The model under review builds one solid part; all positions refer to its coordinate system, in mm. A direction names the side the tool comes from. Round coordinates to 2 decimals unless told otherwise and drop trailing zeros. Order: outer loops, then holes, each group sorted by start corner. A loop starts at its lowest first (then second) coordinate and runs counter-clockwise, first axis right, second up. Notation, with made-up numbers: M 12.5,52 L 30.5,52 A22 cw 30.5,79 Z; hole C -30.75,68.5 d10. An arc over 180 degrees is marked long. Answer as a JSON object with one key per item and string values. Group by question number.
1) To check wall thickness, follow line 1 (Y direction, x = -23.25, z = 0); line 2 (X direction, y = -72, z = -17); line 3 (Z direction, x = -4.5, y = 14.5). State the ranges of each line that lie inside material, in increasing order.
2) Consider section C-C, the plane y = 69.85. Write out the cut boundary in (x, z).
3) Consider section B-B, the plane y = -11.5. Write out the cut boundary in (x, z).
4) Consider section A-A, the plane z = 0. Write out the cut boundary in (x, y).
5) Consider section D-D, the plane x = 10.5. Write out the cut boundary in (y, z), then the cut area to 3 significant figures.
6) For faces 5 (the flat face through (0, 1, -19.05)), 6 (the cylindrical face through (-23.49, 1.42, 23.59)), list the 3-axis set-ups (+Z, -Z, +X, -X, +Y, -Y) from which the entire face can be reached by the end or side of a thin tool; tool diameter is ignored.
7) The part is to be moulded in two halves that separate along Y. For faces 1 (the flat face through (0, -101.6, 22)), 2 (the cylindrical face through (22.27, 54.23, 3.47)), 3 (the cylindrical face through (-22.18, 54.23, 3.47)), 4 (the flat face through (-25.4, 1, 0)), say which applies: +Y half, -Y half, draft (parallel to the pull), parting line (faces both ways), or undercut.
```python
from build123d import *

# Parameters (mm, degrees)
BOSS_EXTRUDE1_DEPTH = 101.6
SKETCH2_R           = 16.002
CUT_EXTRUDE1_DEPTH  = 51.8


with BuildPart() as part:
    # Sketch1 → Boss-Extrude1 (new body, symmetric)
    with BuildSketch(Plane(origin=(0, 0, 0), x_dir=(0, 0, -1), z_dir=(0, 1, 0))):
        with BuildLine():
            Line((-19.05, 25.4), (19.05, 25.4))
            ThreePointArc((19.05, 25.4), (23.540128061, 23.540128061), (25.4, 19.05))
            Line((25.4, 19.05), (25.4, -19.05))
            ThreePointArc((25.4, -19.05), (23.540128061, -23.540128061), (19.05, -25.4))
            Line((19.05, -25.4), (-19.05, -25.4))
            ThreePointArc((-19.05, -25.4), (-23.540128061, -23.540128061), (-25.4, -19.05))
            Line((-25.4, -19.05), (-25.4, 19.05))
            ThreePointArc((-25.4, 19.05), (-23.540128061, 23.540128061), (-19.05, 25.4))
        make_face()
        with BuildLine():
            Line((-16.66875, 19.05), (16.66875, 19.05))
            ThreePointArc((16.66875, 19.05), (18.352548023, 18.352548023), (19.05, 16.66875))
            Line((19.05, 16.66875), (19.05, -16.66875))
            ThreePointArc((19.05, -16.66875), (18.352548023, -18.352548023), (16.66875, -19.05))
            Line((16.66875, -19.05), (-16.66875, -19.05))
            ThreePointArc((-16.66875, -19.05), (-18.352548023, -18.352548023), (-19.05, -16.66875))
            Line((-19.05, -16.66875), (-19.05, 16.66875))
            ThreePointArc((-19.05, 16.66875), (-18.352548023, 18.352548023), (-16.66875, 19.05))
        make_face(mode=Mode.SUBTRACT)
    extrude(amount=BOSS_EXTRUDE1_DEPTH, both=True)

    # Sketch2 → Cut-Extrude1 (cut, through all)
    with BuildSketch(Plane(origin=(25.4, 0, 0), x_dir=(0, 0, -1), z_dir=(1, 0, 0))):
        with Locations((0, 69.85)):
            Circle(SKETCH2_R)
    extrude(amount=-CUT_EXTRUDE1_DEPTH, mode=Mode.SUBTRACT)


solid = part.part
```
Results list:
{
 "1": {"line 1": "-101.6 to 53.85, 85.85 to 101.6", "line 2": "-25.4 to -19.03, 19.03 to 25.4", "line 3": "-25.4 to -19.05, 19.05 to 25.4"},
 "2": {"outline": "M -25.4,-19.05 A6.35 ccw -19.05,-25.4 L 19.05,-25.4 A6.35 ccw 25.4,-19.05 L 25.4,-16 L 19.05,-16 L 19.05,-16.67 A2.38 cw 16.67,-19.05 L -16.67,-19.05 A2.38 cw -19.05,-16.67 L -19.05,-16 L -25.4,-16 Z; M -25.4,16 L -19.05,16 L -19.05,16.67 A2.38 cw -16.67,19.05 L 16.67,19.05 A2.38 cw 19.05,16.67 L 19.05,16 L 25.4,16 L 25.4,19.05 A6.35 ccw 19.05,25.4 L -19.05,25.4 A6.35 ccw -25.4,19.05 Z"},
 "3": {"outline": "M -25.4,-19.05 A6.35 ccw -19.05,-25.4 L 19.05,-25.4 A6.35 ccw 25.4,-19.05 L 25.4,19.05 A6.35 ccw 19.05,25.4 L -19.05,25.4 A6.35 ccw -25.4,19.05 Z; hole M -19.05,-16.67 A2.38 ccw -16.67,-19.05 L 16.67,-19.05 A2.38 ccw 19.05,-16.67 L 19.05,16.67 A2.38 ccw 16.67,19.05 L -16.67,19.05 A2.38 ccw -19.05,16.67 Z"},
 "4": {"outline": "M -25.4,-101.6 L -19.05,-101.6 L -19.05,53.85 L -25.4,53.85 Z; M -25.4,85.85 L -19.05,85.85 L -19.05,101.6 L -25.4,101.6 Z; M 19.05,-101.6 L 25.4,-101.6 L 25.4,53.85 L 19.05,53.85 Z; M 19.05,85.85 L 25.4,85.85 L 25.4,101.6 L 19.05,101.6 Z"},
 "5": {"outline": "M -101.6,-25.4 L 101.6,-25.4 L 101.6,-19.05 L -101.6,-19.05 Z; M -101.6,19.05 L 101.6,19.05 L 101.6,25.4 L -101.6,25.4 Z", "area": "2,580 mm^2"},
 "6": {"face 5": "+Y, -Y", "face 6": "+Z, -X, +Y, -Y"},
 "7": {"face 1": "-Y half", "face 2": "undercut", "face 3": "undercut", "face 4": "draft"}
}
